The model under review builds one solid part; all positions refer to its coordinate system, in mm. Face numbers are marked on the shaded views. A direction names the side the tool comes from. Coordinates: 2 decimals unless noted, no trailing zeros. Loops run counter-clockwise (first coordinate to the right, second up) from the corner with the lowest first, then second, coordinate; pieces in that order, holes last. Notation, with made-up numbers: (-3.5, -15) - (53.5, -15) arc R23 cw to (53.5, -2) - close; hole circle Ø11 at (64, 23.25). An arc over 180 degrees is marked (long way). One line per item, written item: value. Start each with the question number.
1. We need section B-B, the plane z = -3.5. Give the boundary of the cut face in (x, y).
2. To check wall thickness, follow line 1 (Y direction, x = 10, z = 0); line 2 (Y direction, x = 1, z = -0.75); line 3 (Z direction, x = 7.5, y = 1). State the ranges of each line that lie inside material, in increasing order.
3. We need section C-C, the plane x = 5.5. Give the boundary of the cut face in (y, z), then the cut area to 3 significant figures.
4. We need section A-A, the plane x = 4. Give the boundary of the cut face in (y, z), then the cut area to 3 significant figures.
5. We need section D-D, the plane z = 3.75. Give the boundary of the cut face in (x, y).
6. Mouldability with a two-part tool opening along Y and no side actions: class the marked faces 3, 4 and 5 as +Y half, -Y half, draft (parallel to the pull), parting line (faces both ways), or undercut.
7. For the marked faces 1 and 2, list the 3-axis set-ups (+Z, -Z, +X, -X, +Y, -Y) from which the entire face can be reached by the end or side of a thin tool; tool diameter is ignored.
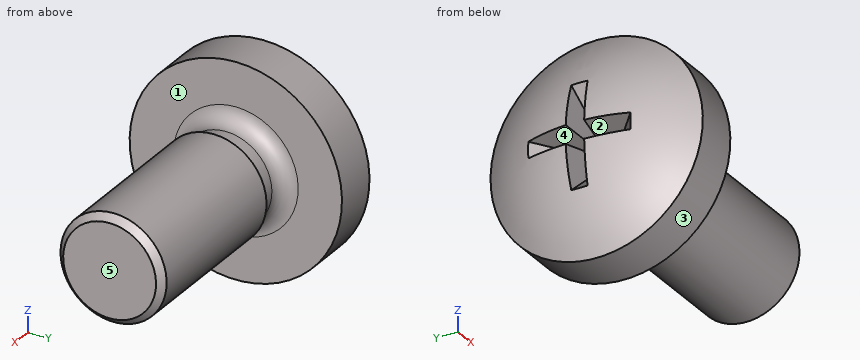
from build123d import *

# Parameters (mm, degrees)
SKETCH_7_W          = 8.1700084
SKETCH_7_H          = 5.261512758
CUT_EXTRUDE_1_DEPTH = 5
CHAMFER_1_SIZE      = 0.25


with BuildPart() as part:
    # 草图2 → Revolve 707 (revolve)
    with BuildSketch(Plane.XY, mode=Mode.PRIVATE) as revolve_707_sk:
        with BuildLine():
            Line((0, 0), (17.1, 0))
            Line((17.1, 0), (17.1, 2))
            Line((17.1, 2), (4.5, 2))
            Line((4.5, 2), (4.232, 1.732))
            Line((4.232, 1.732), (3.718, 1.732))
            ThreePointArc((3.718, 1.732), (3.281008009, 1.913008009), (3.1, 2.35))
            Line((3.1, 2.35), (3.1, 4))
            Line((3.1, 4), (1.376524617, 4))
            ThreePointArc((1.376524617, 4), (0.353757652, 2.115113473), (0, 0))
        make_face()
    revolve(revolve_707_sk.sketch.rotate(Axis((-1.331757704, 0, 0), (1, 0, 0)), 90), axis=Axis((-1.331757704, 0, 0), (1, 0, 0)))

    # 草图3 → 切除-旋转1 (revolve, cut)
    with BuildSketch(Plane.XY, mode=Mode.PRIVATE) as cut_revolve_1_sk:
        Polygon((16.753791204, 2), (17.453791204, 2), (17.1, 1.3938), align=None)
    revolve(cut_revolve_1_sk.sketch.rotate(Axis((-0.242766179, 0, 0), (1, 0, 0)), 90), axis=Axis((-0.242766179, 0, 0), (1, 0, 0)), mode=Mode.SUBTRACT)

    # 草图5 → 切除-放样1 section 0
    with BuildSketch(Plane(origin=(0, 0, 0), x_dir=(0, 0, -1), z_dir=(1, 0, 0)), mode=Mode.PRIVATE) as loft_1_s0:
        with BuildLine():
            Line((0.35, 2.2), (-0.35, 2.2))
            Line((-0.35, 2.2), (-0.35, -2.2))
            Line((-0.35, -2.2), (0.35, -2.2))
            Line((0.35, -2.2), (0.35, 2.2))
        make_face()
    loft_1 = loft([Vertex(2.4, 0, 0), loft_1_s0.sketch], mode=Mode.SUBTRACT)

    # 镜向1: 切除-放样1 across plane
    add(loft_1.mirror(Plane(origin=(0, 0, 0), x_dir=(0, 0.7071067811865462, 0.7071067811865488), z_dir=(0, -0.7071067811865488, 0.7071067811865462))), mode=Mode.SUBTRACT)

    # 草图7 → 切除-拉伸1 (cut, symmetric)
    with BuildSketch(Plane(origin=(0, 0, 0), x_dir=(1, 0, 0), z_dir=(0, 1, 0))):
        with Locations((15.0850042, 0.359536705)):
            Rectangle(SKETCH_7_W, SKETCH_7_H)
    extrude(amount=CUT_EXTRUDE_1_DEPTH, both=True, mode=Mode.SUBTRACT)

    # 倒角1
    chamfer_1_edges = [part.edges().sort_by_distance(p)[0] for p in [
        (11, 0, -2),
    ]]
    chamfer(chamfer_1_edges, length=CHAMFER_1_SIZE)


solid = part.part
Findings below:
1. outline: (1.38, -1.94) - (3.1, -1.94) - (3.1, 1.94) - (1.38, 1.94) arc R5.48 ccw to start
2. line 1: -2 to 2
2. line 2: -3.38 to -0.2, 0.2 to 3.38
2. line 3: -1.73 to 1.73
3. outline: circle Ø4 at (0, 0)
3. area: 12.6 mm2
4. outline: circle Ø3.46 at (0, 0)
4. area: 9.42 mm2
5. outline: (1.38, -1.39) - (3.1, -1.39) - (3.1, 1.39) - (1.38, 1.39) arc R5.31 ccw to start
6. face 3: parting line
6. face 4: undercut
6. face 5: draft
7. face 1: +X
7. face 2: -X
